Geometry check sheet. Reference: the model listing, model coordinates, mm. Face numbers are marked on the shaded views. A direction names the side the tool comes from. Round coordinates to 2 decimals unless told otherwise and drop trailing zeros. Order: outer loops, then holes, each group sorted by start corner. A loop starts at its lowest first (then second) coordinate and runs counter-clockwise, first axis right, second up. Notation, with made-up numbers: M 6,31.25 L 42,31.25 A13 cw 42,50.25 Z; hole C 79,31 d2. An arc over 180 degrees is marked long. Answer as a JSON object with one key per item and string values. Group by question number.
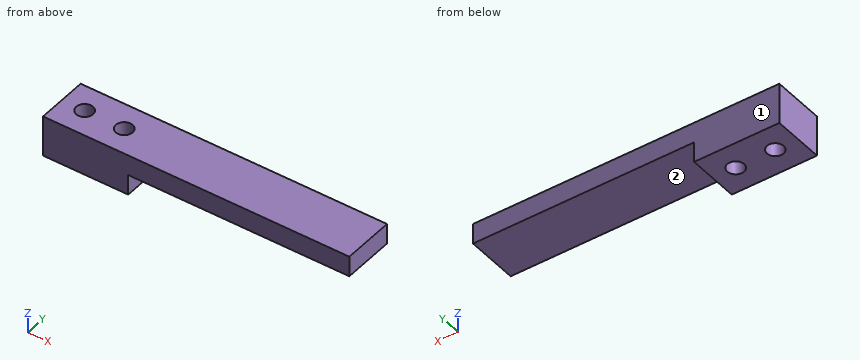
```python
from build123d import *

# Parameters (mm, degrees)
BOSS_EXTRUDE1_DEPTH = 12.7
CUT_EXTRUDE1_DEPTH  = 12.7


with BuildPart() as part:
    # Sketch1 → Boss-Extrude1 (new body)
    with BuildSketch(Plane(origin=(0, 0, 0), x_dir=(1, 0, 0), z_dir=(0, 1, 0))):
        Polygon((-58.57612782, 0), (16.42387218, 0), (16.42387218, 5), (-37.711466165, 5), (-37.711466165, 10), (-58.57612782, 10), align=None)
    extrude(amount=BOSS_EXTRUDE1_DEPTH)

    # Sketch2 → Cut-Extrude1 (cut)
    with BuildSketch(Plane(origin=(0, 0, -10), x_dir=(-1, 0, 0), z_dir=(0, 0, -1))):
        with BuildLine():
            ThreePointArc((41.243796992, 6.35), (43.293796992, 4.3), (45.343796992, 6.35))
            Line((45.343796992, 6.35), (41.243796992, 6.35))
        make_face()
        with BuildLine():
            Line((41.243796992, 6.35), (45.343796992, 6.35))
            ThreePointArc((45.343796992, 6.35), (43.293796992, 8.4), (41.243796992, 6.35))
        make_face()
        with BuildLine():
            ThreePointArc((55.043796992, 6.35), (52.993796992, 8.4), (50.943796992, 6.35))
            Line((50.943796992, 6.35), (55.043796992, 6.35))
        make_face()
        with BuildLine():
            Line((55.043796992, 6.35), (50.943796992, 6.35))
            ThreePointArc((50.943796992, 6.35), (52.993796992, 4.3), (55.043796992, 6.35))
        make_face()
    extrude(amount=-CUT_EXTRUDE1_DEPTH, mode=Mode.SUBTRACT)


solid = part.part
```
1) Go/stop test with flat-tipped pins: P1, Ø3, axis at x = -31, y = 8, coming from the +Z side; P2, Ø6.5, axis at x = -2, y = 6, coming from the -Z side; P3, Ø1.5, axis at y = 4, z = -6.5, coming from the +X side. Record where each tip stops, or that it passes through.
2) Sectioned sample at B-B (x = -53). Record the boundary of the cut face in (y, z), then the cut area to 3 significant figures.
3) Sectioned sample at A-A (y = 6.35). Record the boundary of the cut face in (x, z), then the cut area to 3 significant figures.
4) Sectioned sample at D-D (y = 12). Record the boundary of the cut face in (x, z).
5) Sectioned sample at C-C (z = -7.75). Record the boundary of the cut face in (x, y).
6) Set-up check for the marked faces 1 and 2: record each of +Z, -Z, +X, -X, +Y, -Y from which the full face is reachable in a straight line by a thin tool's end or side.
7) Thickness scan on line 1 along X through (y, z) = (5.5, -2.75); line 2 along Z through (x, y) = (-2, 7.25); line 3 along X through (y, z) = (4.5, -7.5). Record the ranges inside material, lowest first. Write a range as [from, to].
Final values:
{
 "1": {"P1": "stops at z = 0", "P2": "stops at z = -5", "P3": "stops at x = -37.71"},
 "2": {"outline": "M 0,-10 L 4.3,-10 L 4.3,0 L 0,0 Z; M 8.4,-10 L 12.7,-10 L 12.7,0 L 8.4,0 Z", "area": "86.0 mm^2"},
 "3": {"outline": "M -58.58,-10 L -55.04,-10 L -55.04,0 L -58.58,0 Z; M -50.94,-10 L -45.34,-10 L -45.34,0 L -50.94,0 Z; M -41.24,-10 L -37.71,-10 L -37.71,-5 L 16.42,-5 L 16.42,0 L -41.24,0 Z", "area": "397 mm^2"},
 "4": {"outline": "M -58.58,-10 L -37.71,-10 L -37.71,-5 L 16.42,-5 L 16.42,0 L -58.58,0 Z"},
 "5": {"outline": "M -58.58,0 L -37.71,0 L -37.71,12.7 L -58.58,12.7 Z; hole C -52.99,6.35 d4.1; hole C -43.29,6.35 d4.1"},
 "6": {"face 1": "+Z, -Z, +X, -X, +Y", "face 2": "-Z, +X, +Y, -Y"},
 "7": {"line 1": "x = [-58.58, -54.86], [-51.13, -45.16], [-41.43, 16.42]", "line 2": "z = [-5, 0]", "line 3": "x = [-58.58, -53.88], [-52.11, -44.18], [-42.41, -37.71]"}
}
